Geometry: final body of the model. Coordinates: model frame, mm. A direction names the side the tool comes from. Round coordinates to 2 decimals unless told otherwise and drop trailing zeros. Loops run counter-clockwise (first coordinate to the right, second up) from the corner with the lowest first, then second, coordinate; pieces in that order, holes last. Notation, with made-up numbers: (-37.5, 39.5) -> (-7.5, 39.5) arc R23 ccw to (-7.5, 66.5) -> close; hole circle Ø7 at (54, 51). An arc over 180 degrees is marked (long way). Answer in a Markdown table with one row per item.
Autodesk Inventor part; units mm, degrees
ref_plane "YZ Plane" through (0, 0, 0) normal (1, 0, 0) x (0, 1, 0)
ref_plane "XZ Plane" through (0, 0, 0) normal (0, 1, 0) x (-1, 0, 0)
ref_plane "XY Plane" through (0, 0, 0) normal (0, 0, 1) x (1, 0, 0)
sketch "Sketch1" plane through (0, 0, 0) normal (0, 1, 0) x (-1, 0, 0)
  line L0 (0, 25.4) -> (685.8, 25.4)
  line L1 (0, 0) -> (685.8, 0)
  line L2 (685.8, 0) -> (685.8, 25.4)
  line L3 (0, 0) -> (-50.8, 0)
  line L4 (0, 25.4) -> (-50.8, 25.4)
  line L5 (-50.8, 25.4) -> (-50.8, 0)
  dimension "d0" = 25.4
  dimension "d1" = 685.8
  dimension "d20" = 50.8
extrude "Extrusion1" add sketch "Sketch1" along normal blind 50.8
sketch "Sketch6" plane through (50.8, 0, 25.4) normal (1, 0, 0) x (0, 0, -1)
  line L0 (0, 50.8) -> (0, 0)
  line L1 (0, 0) -> (25.4, 0)
  line L2 (25.4, 0) -> (25.4, 50.8)
  line L3 (25.4, 50.8) -> (0, 50.8)
  line L4 (25.4, 50.8) -> (0, 50.8)
  line L5 (3.1242, 47.6758) -> (3.1242, 3.1242)
  line L6 (3.1242, 3.1242) -> (22.2758, 3.1242)
  line L7 (22.2758, 3.1242) -> (22.2758, 47.6758)
  line L8 (22.2758, 47.6758) -> (3.1242, 47.6758)
  dimension "d21" = 3.1242
extrude "Extrusion4" cut sketch "Sketch6" against normal blind 736.6 contours L8 L7 L6 L5
sketch "Sketch7" plane through (0, 50.8, 0) normal (0, 1, 0) x (1, 0, 0)
  point P0 (0, 0)
  point P1 (0, -12.7)
properties part number "Arm" material "Aluminum 6061"
Item 1: Pin query (flat end, axial travel): pin 1 Ø12 at (x, y) = (-249, 9) entering from -Z; pin 2 Ø1 at (y, z) = (35.5, 4.5) entering from -X. Return the tip coordinate at first contact, or that it passes through.
Answer:
| item | result |
|---|---|
| pin 1 | stops at z = 0 |
| pin 2 | passes through |
Item 2: Reachability of faces 4 (the face through (-312, 26, 22.276)), 5 (the face through (-312, 25, 25.4)) from +Z, -Z, +X, -X, +Y, -Y: full face, straight path, thin tool, end or side. Return the list, or none.
Answer:
| item | result |
|---|---|
| face 4 | +X, -X |
| face 5 | +Z, +X, -X, +Y, -Y |
Item 3: Cut plane A-A (y = 27.5). Output: boundary loops of the cut face in (x, z).
Answer:
| item | result |
|---|---|
| outline | (-685.8, 0) -> (50.8, 0) -> (50.8, 3.12) -> (-685.8, 3.12) -> close; (-685.8, 22.28) -> (50.8, 22.28) -> (50.8, 25.4) -> (-685.8, 25.4) -> close |
Item 4: Line query: probe 1 along Z at (x, y) = (-445, 21.5); probe 2 along Y at (x, z) = (-536.5, 14.25). Output: solid intervals per line, ascending. Write a range as [from, to].
Answer:
| item | result |
|---|---|
| probe 1 | z = [0, 3.12], [22.28, 25.4] |
| probe 2 | y = [0, 3.12], [47.68, 50.8] |
Item 5: Cut plane C-C (x = -444.5). Output: boundary loops of the cut face in (y, z).
Answer:
| item | result |
|---|---|
| outline | (0, 0) -> (50.8, 0) -> (50.8, 25.4) -> (0, 25.4) -> close; hole (3.12, 3.12) -> (47.68, 3.12) -> (47.68, 22.28) -> (3.12, 22.28) -> close |
Item 6: Cut plane B-B (z = 7.75). Output: boundary loops of the cut face in (x, y), then the cut area to 3 significant figures.
Answer:
| item | result |
|---|---|
| outline | (-685.8, 0) -> (50.8, 0) -> (50.8, 3.12) -> (-685.8, 3.12) -> close; (-685.8, 47.68) -> (50.8, 47.68) -> (50.8, 50.8) -> (-685.8, 50.8) -> close |
| area | 4,600 mm² |
Item 7: Draft query along Y for faces 1 (the face through (-312, 47.676, 13)), 2 (the face through (-312, 50.8, 13)), 3 (the face through (-685.8, 27, 2)). Return one class per face: pulls with the +Y half, pulls with the -Y half, needs draft (parallel to the pull), parting line crosses it, or undercut.
Answer:
| item | result |
|---|---|
| face 1 | undercut |
| face 2 | pulls with the +Y half |
| face 3 | needs draft |
